Autodesk Inventor part; units mm, degrees
ref_plane "YZ Plane" through (0, 0, 0) normal (1, 0, 0) x (0, 1, 0)
ref_plane "XZ Plane" through (0, 0, 0) normal (0, 1, 0) x (-1, 0, 0)
ref_plane "XY Plane" through (0, 0, 0) normal (0, 0, 1) x (1, 0, 0)
sketch "Sketch1" plane through (0, 0, 0) normal (0, 0, 1) x (1, 0, 0)
  line L0 (20, 0) -> (133, 0)
  line L1 (153, 8) -> (153, 22)
  line L2 (133, 30) -> (20, 30)
  line L3 (0, 22) -> (0, 8)
  line L4 (150, 25) -> (135, 25)
  line L5 (133, 27) -> (133, 30)
  line L6 (3, 25) -> (18, 25)
  line L7 (20, 27) -> (20, 30)
  line L8 (3, 5) -> (18, 5)
  line L9 (20, 3) -> (20, 0)
  arc A0 (18, 25) -> (20, 27) centre (18, 27) ccw
  arc A1 (20, 3) -> (18, 5) centre (18, 3) ccw
  arc A2 (133, 27) -> (135, 25) centre (135, 27) ccw
  line L10 (150, 5) -> (135, 5)
  line L11 (0, 22) -> (3, 22)
  line L12 (3, 22) -> (3, 25)
  line L13 (0, 8) -> (3, 8)
  line L14 (3, 8) -> (3, 5)
  line L15 (150, 25) -> (150, 22)
  line L16 (150, 22) -> (153, 22)
  line L17 (150, 5) -> (150, 8)
  line L18 (150, 8) -> (153, 8)
  line L19 (133, 0) -> (133, 3)
  arc A3 (135, 5) -> (133, 3) centre (135, 3) ccw
  point P0 (0, 0)
  point P1 (133, 25)
  point P2 (20, 25)
  point P3 (20, 5)
  point P4 (133, 5)
  dimension "d31" = 5
  dimension "d33" = 5
  dimension "d36" = 5
  dimension "d37" = 113
  dimension "d39" = 2
  dimension "d46" = 2
  dimension "d59" = 3
  dimension "d60" = 3
  dimension "d61" = 3
  dimension "d62" = 3
  dimension "d64" = 14
  dimension "d65" = 20
  dimension "d66" = 3
  dimension "d67" = 3
  dimension "d68" = 14
  dimension "d70" = 3
  dimension "d75" = 2
  dimension "d76" = 20
  dimension "d88" = 20
  dimension "d89" = 20
extrude "Extrusion1" add sketch "Sketch1" along normal blind 3
sketch "Sketch3" plane through (0, 0, 3) normal (0, 0, 1) x (1, 0, 0)
  circle A0 centre (76.5, 15) radius 9
  line L0 (20, 30) -> (133, 30)
  line L1 (153, 8) -> (153, 22)
  point P0 (0, 0)
  point P1 (2, 30)
  point P2 (151, 30)
  point P3 (153, 2)
  point P4 (153, 28)
  point P5 (27, 30)
  point P6 (126, 30)
  point P7 (153, 7)
  point P8 (153, 23)
  dimension "d24" = 18
  dimension "d25" = 15
  dimension "d26" = 76.5
extrude "Extrusion3" cut sketch "Sketch3" against normal through all
sketch "Sketch4" plane through (0, 0, 3) normal (0, 0, 1) x (1, 0, 0)
  circle A0 centre (26.5, -3.5) radius 3
  circle A1 centre (76.5, 15) radius 9
  line L0 (20, 0) -> (55, 0)
  line L1 (33, -10) -> (20, -10)
  line L2 (20, -10) -> (20, 0)
  line L3 (76.5, 0) -> (76.5, 30) construction
  line L4 (133, 30) -> (20, 30) construction
  circle A2 centre (126.5, -3.5) radius 3
  line L5 (133, 0) -> (98, 0)
  line L6 (120, -10) -> (133, -10)
  line L7 (133, -10) -> (133, 0)
  line L8 (33, -10) -> (55, 0)
  line L9 (120, -10) -> (98, 0)
  line L10 (55, 0) -> (59.5455, -10)
  line L11 (98, 0) -> (93.4545, -10)
  line L12 (93.4545, -10) -> (59.5455, -10)
  line L13 (55, 0) -> (98, 0)
  line L14 (133, 0) -> (20, 0)
  point P0 (0, 0)
  point P1 (126, 30)
  point P2 (27, 30)
  dimension "d40" = 6
  dimension "d41" = 50
  dimension "d48" = 10
  dimension "d49" = 13
  dimension "d50" = 3.5
  dimension "d54" = 35
  dimension "d55" = 35
extrude "Extrusion6" add sketch "Sketch4" against normal blind 3 contours L5 L7 L6 L9 | L13 L11 L12 L10 | L0 L8 L1 L2
sketch "Sketch7" plane through (0, 0, 3) normal (0, 0, 1) x (1, 0, 0)
  line L0 (20, 30) -> (20, 35)
  line L1 (20, 35) -> (47.7273, 35)
  line L2 (47.7273, 35) -> (50, 30)
  line L3 (20, 30) -> (133, 30)
  line L4 (50, 30) -> (61, 35)
  line L5 (55, 0) -> (59.5455, -10)
  line L6 (33, -10) -> (55, 0)
  line L7 (133, 30) -> (133, 35)
  line L8 (133, 35) -> (105.2727, 35)
  line L9 (105.2727, 35) -> (103, 30)
  line L10 (103, 30) -> (92, 35)
  line L11 (92, 35) -> (61, 35)
  line L12 (98, 0) -> (120, -10)
  line L13 (93.4545, -10) -> (98, 0)
  point P0 (0, 0)
  point P1 (57.069, -4.5518)
  point P2 (58.2132, -7.069)
  point P3 (33.986, -9.5518)
  point P4 (50.4482, -2.069)
  point P5 (102.5518, -2.069)
  point P6 (119.014, -9.5518)
  point P7 (94.7868, -7.069)
  point P8 (95.931, -4.5518)
  dimension "d80" = 5
  dimension "d81" = 30
  dimension "d82" = 30
extrude "Extrusion7" add sketch "Sketch7" against normal blind 3
fillet "Fillet4" radius 5 2 edges at (50, 30, 1.5) (103, 30, 1.5)
fillet "Fillet5" radius 5 2 edges at (55, 0, 1.5) (98, 0, 1.5)
fillet "Fillet6" radius 5 12 edges at (20, -10, 1.5) (20, 35, 1.5) (47.7273, 35, 1.5) (61, 35, 1.5) (92, 35, 1.5) (105.2727, 35, 1.5) (133, 35, 1.5) (133, -10, 1.5) (120, -10, 1.5) (93.4545, -10, 1.5) (59.5455, -10, 1.5) (33, -10, 1.5)
sketch "Sketch10" plane through (0, 0, 0) normal (0, 0, -1) x (-1, 0, 0)
  line L0 (-123.5, 2.5) -> (-29.5, 2.5)
  line L1 (-26.5, 5.5) -> (-26.5, 24.5)
  line L2 (-29.5, 27.5) -> (-123.5, 27.5)
  line L3 (-126.5, 24.5) -> (-126.5, 5.5)
  circle A0 centre (-76.5, 15) radius 9
  line L4 (-126.5, 2.5) -> (-26.5, 27.5) construction
  line L5 (-26.5, 2.5) -> (-126.5, 27.5) construction
  arc A1 (-123.5, 27.5) -> (-126.5, 24.5) centre (-123.5, 24.5) ccw
  arc A2 (-26.5, 24.5) -> (-29.5, 27.5) centre (-29.5, 24.5) ccw
  arc A3 (-29.5, 2.5) -> (-26.5, 5.5) centre (-29.5, 5.5) ccw
  arc A4 (-126.5, 5.5) -> (-123.5, 2.5) centre (-123.5, 5.5) ccw
  point P0 (0, 0)
  dimension "d90" = 25
  dimension "d91" = 100
  dimension "d92" = 3
extrude "Extrusion8" cut sketch "Sketch10" against normal through all
properties part number "27030914FacePlate"
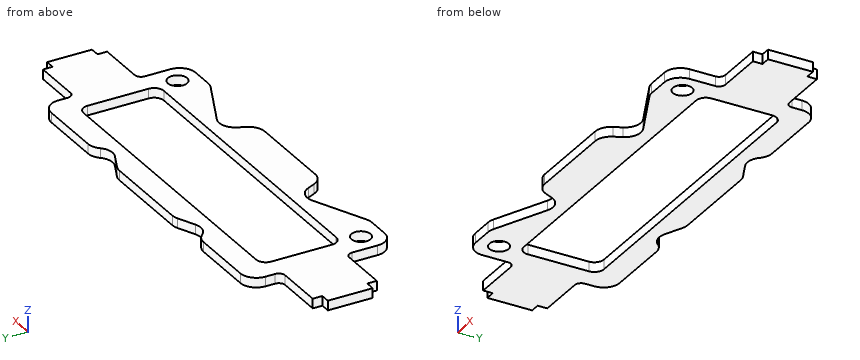
Check sheet for the modelled part. Datum: model origin and axes. Units: mm. Give positions to 0.01 mm unless a question says otherwise; leave off trailing zeros. Write each loop counter-clockwise with the first axis right and the second up, starting at its lowest first coordinate (ties: lowest second). Pieces come first, ordered by that corner, then holes. Notation, with made-up numbers: M 22.25,29 L 81.25,29 A9 ccw 81.25,38 Z; hole C 21,-6.75 d9. An arc over 180 degrees is marked long. Use one line per item in the form item = value.
(1) Depth check by flat-ended pin: P1, Ø1.5, axis at y = 6.5, z = 1.5, coming from the +X side; P2, Ø1.5, axis at y = 29, z = 2, coming from the +X side; P3, Ø0.9, axis at x = 12, z = 2, coming from the -Y side; P4, Ø5, axis at x = 26.5, y = -3.5, coming from the -Z side. Enter the tip coordinate at first touch or a pass-through.
Answer block:
P1 = 150
P2 = 133
P3 = 5
P4 = through
(2) Section check B-B on x = 67.5. Record the boundary of the cut face in (y, z).
Answer block:
outline = M -10,0 L 2.5,0 L 2.5,3 L -10,3 Z; M 27.5,0 L 35,0 L 35,3 L 27.5,3 Z
(3) Material ranges on line 1 along X through (y, z) = (33, 0.45); line 2 along X through (y, z) = (16, 2.8); line 3 along Y through (x, z) = (65.5, 1.95), recorded low to high.
Answer block:
line_1 = 21 to 49.03, 56.6 to 96.4, 103.97 to 132
line_2 = 0 to 26.5, 126.5 to 153
line_3 = -10 to 2.5, 27.5 to 35
(4) Section check C-C on x = 141. Record the boundary of the cut face in (y, z).
Answer block:
outline = M 5,0 L 25,0 L 25,3 L 5,3 Z
(5) Section check D-D on z = 2.15. State how many separate pieces and enclosed holes the cut face has, plus the area to 3 significant figures.
Answer block:
separate_pieces = 1
enclosed_holes = 3
area = 2,970 mm2
(6) Section check A-A on y = 11.5. Record the boundary of the cut face in (x, z), plus the area to 3 significant figures.
Answer block:
outline = M 0,0 L 26.5,0 L 26.5,3 L 0,3 Z; M 126.5,0 L 153,0 L 153,3 L 126.5,3 Z
area = 159 mm2
